The model under review builds one solid part; all positions refer to its coordinate system, in mm. Face numbers are marked on the shaded views. A direction names the side the tool comes from. Coordinates: 2 decimals unless noted, no trailing zeros. Loops run counter-clockwise (first coordinate to the right, second up) from the corner with the lowest first, then second, coordinate; pieces in that order, holes last. Notation, with made-up numbers: M 46,32.25 L 95,32.25 A24 cw 95,49.25 Z; hole C 79,-22.5 d10. An arc over 180 degrees is marked long. Write item = value, one per line. Start each with the question number.
Q1. Clearance check with flat-ended pins moving along their axes: pin 1 Ø12 at (y, z) = (10, 11.5) entering from +X; pin 2 Ø10 at (y, z) = (2.5, -32.5) entering from -X; pin 3 Ø1.5 at (x, y) = (-40.5, 12) entering from +Z; pin 4 Ø8 at (y, z) = (10, 10) entering from -X. State where each tip first meets the part, or that it passes through.
Q2. We need section A-A on x = -27. Give the boundary of the cut face in (y, z), and give its area (3 significant figures).
Q3. For the marked faces 1, 2, 3 and 4, list the 3-axis set-ups (+Z, -Z, +X, -X, +Y, -Y) from which the entire face can be reached by the end or side of a thin tool; tool diameter is ignored.
Q4. Wall thickness on probe 1 along Y at (x, z) = (-2, 10); probe 2 along X at (y, z) = (12.25, 3); probe 3 along X at (y, z) = (6.75, -62): over which ranges is each line inside the solid? List them lowest first.
Q5. We need section B-B on y = 10. Give the boundary of the cut face in (x, z), and give its area (3 significant figures).
Q6. We need section C-C on z = 10. Give the boundary of the cut face in (x, y).
Q7. Mouldability with a two-part tool opening along Z and no side actions: class the marked faces 5, 6 and 7 as released by +Z, released by -Z, zero draft, split by the parting line, or undercut.
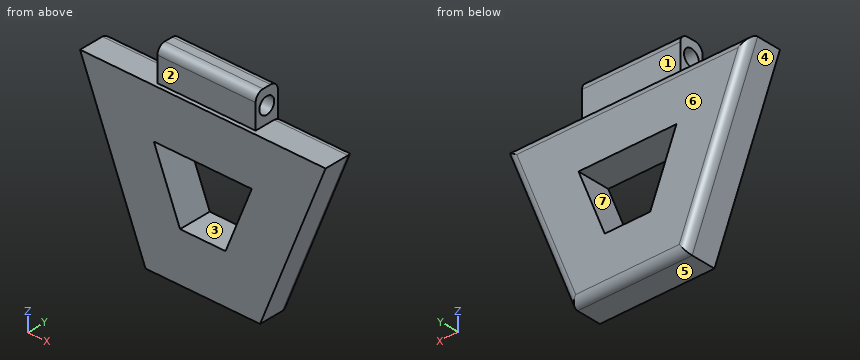
from build123d import *

# Parameters (mm, degrees)
BOSS_EXTRUDE1_DEPTH = 20
SKETCH2_W           = 60
SKETCH2_H           = 15
BOSS_EXTRUDE2_DEPTH = 20
SKETCH3_R           = 5
CUT_EXTRUDE1_DEPTH  = 147.372811683
FILLET1_R           = 5


with BuildPart() as part:
    # Sketch1 → Boss-Extrude1 (new body)
    with BuildSketch(Plane(origin=(0, 0, 0), x_dir=(1, 0, 0), z_dir=(0, 1, 0))):
        Polygon((-35, 100), (35, 100), (75, 0), (-75, 0), align=None)
        Polygon((-13.9, 70), (13.9, 70), (29.9, 30), (-29.9, 30), align=None, mode=Mode.SUBTRACT)
    extrude(amount=BOSS_EXTRUDE1_DEPTH)

    # Sketch2 → Boss-Extrude2 (add)
    with BuildSketch(Plane.XY):
        with Locations((0, 10)):
            Rectangle(SKETCH2_W, SKETCH2_H)
    extrude(amount=BOSS_EXTRUDE2_DEPTH)

    # Sketch3 → Cut-Extrude1 (cut, through all)
    with BuildSketch(Plane(origin=(30, 0, 0), x_dir=(0, 0, -1), z_dir=(1, 0, 0))):
        with Locations((-10, 10)):
            Circle(SKETCH3_R)
    extrude(amount=-CUT_EXTRUDE1_DEPTH, mode=Mode.SUBTRACT)

    # Fillet1
    # the kernel refuses this fillet: 5 mm, written as the material it takes off along each edge
    with BuildSketch(Plane(origin=(87.5, 20, 0), x_dir=(0, 0, -1), z_dir=(-1, 0, 0))) as fillet1_piece_1_section:
        with BuildLine():
            CenterArc((FILLET1_R, FILLET1_R), FILLET1_R, 180, 90)
            Line((0, FILLET1_R), (0, 0))
            Line((0, 0), (FILLET1_R, 0))
        make_face()
    fillet1_piece_1 = extrude(amount=175, mode=Mode.PRIVATE)
    fillet1_piece_1 = split(fillet1_piece_1, bisect_by=Plane(origin=(30, 19.178041178, -1.2756003), z_dir=(1, 0, 0)), keep=Keep.TOP, mode=Mode.PRIVATE)
    fillet1_piece_1 = split(fillet1_piece_1, bisect_by=Plane(origin=(58.75, 17.5, -1.2756003), z_dir=(0, 1, 0)), keep=Keep.TOP, mode=Mode.PRIVATE)
    add(fillet1_piece_1, mode=Mode.SUBTRACT)
    with BuildSketch(Plane(origin=(87.5, 20, 0), x_dir=(0, 0, -1), z_dir=(-1, 0, 0))) as fillet1_piece_2_section:
        with BuildLine():
            CenterArc((FILLET1_R, FILLET1_R), FILLET1_R, 180, 90)
            Line((0, FILLET1_R), (0, 0))
            Line((0, 0), (FILLET1_R, 0))
        make_face()
    fillet1_piece_2 = extrude(amount=175, mode=Mode.PRIVATE)
    fillet1_piece_2 = split(fillet1_piece_2, bisect_by=Plane(origin=(30, 16.683746077, -0.120041908), z_dir=(1, 0, 0)), keep=Keep.TOP, mode=Mode.PRIVATE)
    fillet1_piece_2 = split(fillet1_piece_2, bisect_by=Plane(origin=(58.75, 17.5, -0.120041908), z_dir=(0, -1, 0)), keep=Keep.TOP, mode=Mode.PRIVATE)
    add(fillet1_piece_2, mode=Mode.SUBTRACT)
    with BuildSketch(Plane(origin=(87.5, 20, 0), x_dir=(0, 0, -1), z_dir=(-1, 0, 0))) as fillet1_piece_3_section:
        with BuildLine():
            CenterArc((FILLET1_R, FILLET1_R), FILLET1_R, 180, 90)
            Line((0, FILLET1_R), (0, 0))
            Line((0, 0), (FILLET1_R, 0))
        make_face()
    fillet1_piece_3 = extrude(amount=175, mode=Mode.PRIVATE)
    fillet1_piece_3 = split(fillet1_piece_3, bisect_by=Plane(origin=(-30, 19.178041178, -1.2756003), z_dir=(1, 0, 0)), keep=Keep.TOP, mode=Mode.PRIVATE)
    fillet1_piece_3 = split(fillet1_piece_3, bisect_by=Plane(origin=(30, 19.178041178, -1.2756003), z_dir=(-1, 0, 0)), keep=Keep.TOP, mode=Mode.PRIVATE)
    fillet1_piece_3 = split(fillet1_piece_3, bisect_by=Plane(origin=(0, 17.5, -1.2756003), z_dir=(0, 1, 0)), keep=Keep.TOP, mode=Mode.PRIVATE)
    add(fillet1_piece_3, mode=Mode.SUBTRACT)
    with BuildSketch(Plane(origin=(87.5, 20, 0), x_dir=(0, 0, -1), z_dir=(-1, 0, 0))) as fillet1_piece_4_section:
        with BuildLine():
            CenterArc((FILLET1_R, FILLET1_R), FILLET1_R, 180, 90)
            Line((0, FILLET1_R), (0, 0))
            Line((0, 0), (FILLET1_R, 0))
        make_face()
    fillet1_piece_4 = extrude(amount=175, mode=Mode.PRIVATE)
    fillet1_piece_4 = split(fillet1_piece_4, bisect_by=Plane(origin=(-30, 19.178041178, -1.2756003), z_dir=(-1, 0, 0)), keep=Keep.TOP, mode=Mode.PRIVATE)
    fillet1_piece_4 = split(fillet1_piece_4, bisect_by=Plane(origin=(-58.75, 17.5, -1.2756003), z_dir=(0, 1, 0)), keep=Keep.TOP, mode=Mode.PRIVATE)
    add(fillet1_piece_4, mode=Mode.SUBTRACT)
    with BuildSketch(Plane(origin=(87.5, 20, 0), x_dir=(0, 0, -1), z_dir=(-1, 0, 0))) as fillet1_piece_5_section:
        with BuildLine():
            CenterArc((FILLET1_R, FILLET1_R), FILLET1_R, 180, 90)
            Line((0, FILLET1_R), (0, 0))
            Line((0, 0), (FILLET1_R, 0))
        make_face()
    fillet1_piece_5 = extrude(amount=175, mode=Mode.PRIVATE)
    fillet1_piece_5 = split(fillet1_piece_5, bisect_by=Plane(origin=(-30, 16.683746077, -0.120041908), z_dir=(-1, 0, 0)), keep=Keep.TOP, mode=Mode.PRIVATE)
    fillet1_piece_5 = split(fillet1_piece_5, bisect_by=Plane(origin=(-58.75, 17.5, -0.120041908), z_dir=(0, -1, 0)), keep=Keep.TOP, mode=Mode.PRIVATE)
    add(fillet1_piece_5, mode=Mode.SUBTRACT)
    with BuildSketch(Plane(origin=(-79.642383454, 20, 11.605958636), x_dir=(0, -1, 0), z_dir=(0.37139067635410355, 0, -0.9284766908852595)), Plane(origin=(30.357616546, 20, -111.605958636), x_dir=(0, -1, 0), z_dir=(0.37139067635410383, 0, 0.9284766908852593))) as fillet1_piece_6:
        with BuildLine():
            CenterArc((FILLET1_R, -FILLET1_R), FILLET1_R, 90, 90)
            Line((0, -FILLET1_R), (0, 0))
            Line((0, 0), (FILLET1_R, 0))
        make_face()
    extrude(amount=132.703296143, mode=Mode.SUBTRACT)
    with BuildSketch(Plane(origin=(-47.5, 20, -100), x_dir=(0, -1, 0), z_dir=(1, 0, 0))) as fillet1_piece_7:
        with BuildLine():
            CenterArc((FILLET1_R, -FILLET1_R), FILLET1_R, 90, 90)
            Line((0, -FILLET1_R), (0, 0))
            Line((0, 0), (FILLET1_R, 0))
        make_face()
    extrude(amount=95, mode=Mode.SUBTRACT)
    with BuildSketch(Plane(origin=(42.5, 2.5, 20), x_dir=(0, 0, -1), z_dir=(-1, 0, 0)), Plane(origin=(-42.5, 17.5, 20), x_dir=(0, 0, -1), z_dir=(1, 0, 0))) as fillet1_piece_8:
        with BuildLine():
            CenterArc((FILLET1_R, -FILLET1_R), FILLET1_R, 90, 90)
            Line((0, -FILLET1_R), (0, 0))
            Line((0, 0), (FILLET1_R, 0))
        make_face()
    extrude(amount=85, mode=Mode.SUBTRACT)


solid = part.part
Returned:
q1.pin_1 = 30
q1.pin_2 = -64
q1.pin_3 = 0
q1.pin_4 = through
q2.outline = M 0,-100 L 15,-100 A5 ccw 20,-95 L 20,-37.25 L 0,-37.25 Z; M 0,-30 L 20,-30 L 20,-5 A5 ccw 17.5,-0.67 L 17.5,15 A5 ccw 12.5,20 L 7.5,20 A5 ccw 2.5,15 L 2.5,0 L 0,0 Z; hole C 10,10 d10
q2.area = 2,060 mm^2
q3.face_1 = +Z, +X, -X, +Y
q3.face_2 = +Z, +X, -X, -Y
q3.face_3 = +Y, -Y
q3.face_4 = -Z, -X, +Y, -Y
q4.probe_1 = 2.5 to 5, 15 to 17.5
q4.probe_2 = -30 to 30
q4.probe_3 = -50.2 to -17.1, 17.1 to 50.2
q5.outline = M -75,0 L -35,-100 L 35,-100 L 75,0 L 30,0 L 30,5 L -30,5 L -30,0 Z; M -30,15 L 30,15 L 30,20 L -30,20 Z; hole M -29.9,-30 L -13.9,-70 L 13.9,-70 L 29.9,-30 Z
q5.area = 9,850 mm^2
q6.outline = M -30,2.5 L 30,2.5 L 30,5 L -30,5 Z; M -30,15 L 30,15 L 30,17.5 L -30,17.5 Z
q7.face_5 = released by -Z
q7.face_6 = zero draft
q7.face_7 = undercut
